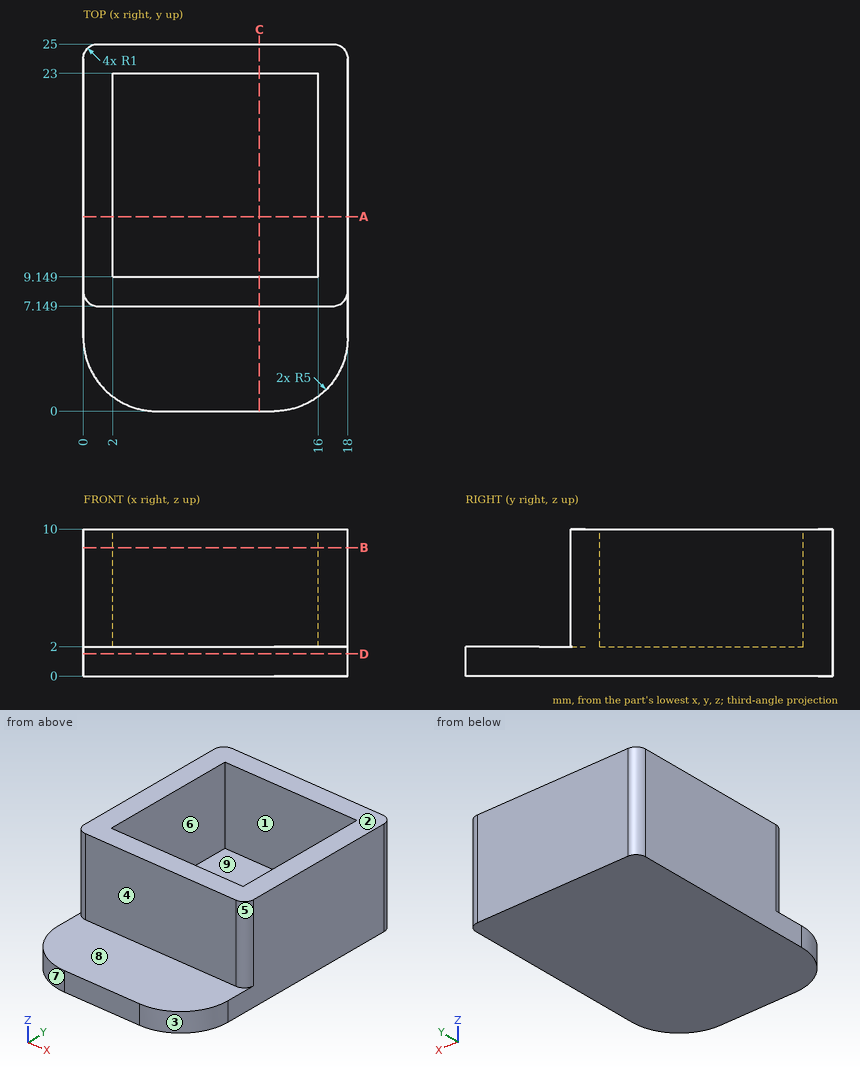
Drawing for the job (mm, zero at the part's lowest x, y, z). A direction names the side the tool comes from. Round coordinates to 2 decimals unless told otherwise and drop trailing zeros. Write each loop counter-clockwise with the first axis right and the second up, starting at its lowest first coordinate (ties: lowest second). Pieces come first, ordered by that corner, then holes. Notation, with made-up numbers: M -8.5,17 L -2.5,17 A24 cw -2.5,54 Z; hole C 52.5,80 d4. An arc over 180 degrees is marked long. Answer as a JSON object with one key per item and string values. Group by question number.
(1) Cut at B-B (z = 8.75). Give the cut face in (x, y).
(2) Which spindle directions (+Z, -Z, +X, -X, +Y, -Y) get a long thin tool onto all of the face, cutting with end or side? Do the marked faces 1, 2, 3, 4 and 5. Say none if no direction does.
(3) Cut at C-C (x = 12). Give the cut face in (y, z), and give its area (3 significant figures).
(4) Cut at D-D (z = 1.5). Give the cut face in (x, y).
(5) Cut at A-A (y = 13.25). Give the cut face in (x, z), and give its area (3 significant figures).
(6) Mould opens along X. For the marked faces 6, 7, 8 and 9 say: pulls with the +X half, pulls with the -X half, needs draft (parallel to the pull), parting line crosses it, or undercut.
(7) Drill centre lines: L1, parallel to X at y = 14, z = 8; L2, parallel to Y at x = 6.5, z = 3; L3, parallel to Z at x = 5.5, y = 2.75. Where is each one in solid material? Low to high.
(8) Flat gauge pins, fed straight in: pin 1 (7 mm diameter, centred on x = 9.5, y = 18, fed in from +Z); pin 2 (3 mm diameter, centred on x = 4, y = 6.5, fed in from +Z); pin 3 (4 mm diameter, centred on x = 7, z = 6.5, fed in from -Y). Where does each tip first touch, or does it go through?
Responses:
{
 "1": {"outline": "M 0,8.15 A1 ccw 1,7.15 L 17,7.15 A1 ccw 18,8.15 L 18,24 A1 ccw 17,25 L 1,25 A1 ccw 0,24 Z; hole M 2,9.15 L 16,9.15 L 16,23 L 2,23 Z"},
 "2": {"face 1": "+Z", "face 2": "+Z, +X, -X, +Y, -Y", "face 3": "+Z, -Z, +X, -Y", "face 4": "+Z, +X, -X, -Y", "face 5": "+Z, +X, -Y"},
 "3": {"outline": "M 0,0 L 25,0 L 25,10 L 23,10 L 23,2 L 9.15,2 L 9.15,10 L 7.15,10 L 7.15,2 L 0,2 Z", "area": "82.0 mm2"},
 "4": {"outline": "M 0,5 A5 ccw 5,0 L 13,0 A5 ccw 18,5 L 18,24 A1 ccw 17,25 L 1,25 A1 ccw 0,24 Z"},
 "5": {"outline": "M 0,0 L 18,0 L 18,10 L 16,10 L 16,2 L 2,2 L 2,10 L 0,10 Z", "area": "68.0 mm2"},
 "6": {"face 6": "undercut", "face 7": "pulls with the -X half", "face 8": "needs draft", "face 9": "undercut"},
 "7": {"L1": "x = 0 to 2, 16 to 18", "L2": "y = 7.15 to 9.15, 23 to 25", "L3": "z = 0 to 2"},
 "8": {"pin 1": "stops at z = 2", "pin 2": "stops at z = 10", "pin 3": "stops at y = 7.15"}
}
